```python
from build123d import *

# Parameters (mm, degrees)
SKETCH1_R           = 57.5
SKETCH1_R_2         = 39.25
BOSS_EXTRUDE1_DEPTH = 10
SKETCH2_R           = 1.75
CUT_EXTRUDE1_DEPTH  = 17
SKETCH3_R           = 47
CUT_EXTRUDE2_DEPTH  = 0.75
SKETCH5_R           = 2
CUT_EXTRUDE3_DEPTH  = 5
SKETCH6_R           = 39.25
SKETCH6_R_2         = 35
BOSS_EXTRUDE2_DEPTH = 2


with BuildPart() as part:
    # Sketch1 → Boss-Extrude1 (new body)
    with BuildSketch(Plane(origin=(0, 0, 0), x_dir=(1, 0, 0), z_dir=(0, 1, 0))):
        with Locations(Location((0, 0, 0), (0, 0, 270))):
            Circle(SKETCH1_R)
        with Locations(Location((0, 0, 0), (0, 0, 270))):
            Circle(SKETCH1_R_2, mode=Mode.SUBTRACT)
    extrude(amount=BOSS_EXTRUDE1_DEPTH)

    # Sketch2 → Cut-Extrude1 (cut)
    with BuildSketch(Plane(origin=(0, 10, 0), x_dir=(1, 0, 0), z_dir=(0, 1, 0))):
        with Locations(Location((0, 54, 0), (0, 0, 270))):
            Circle(SKETCH2_R)
        with Locations(Location((20.664905348, 49.889494756, 0), (0, 0, 270))):
            Circle(SKETCH2_R)
        with Locations(Location((38.183766184, 38.183766184, 0), (0, 0, 270))):
            Circle(SKETCH2_R)
        with Locations(Location((49.889494756, 20.664905348, 0), (0, 0, 270))):
            Circle(SKETCH2_R)
        with Locations(Location((54, 0, 0), (0, 0, 270))):
            Circle(SKETCH2_R)
        with Locations(Location((49.889494756, -20.664905348, 0), (0, 0, 270))):
            Circle(SKETCH2_R)
        with Locations(Location((38.183766184, -38.183766184, 0), (0, 0, 270))):
            Circle(SKETCH2_R)
        with Locations(Location((20.664905348, -49.889494756, 0), (0, 0, 270))):
            Circle(SKETCH2_R)
        with Locations(Location((0, -54, 0), (0, 0, 270))):
            Circle(SKETCH2_R)
        with Locations(Location((-20.664905348, -49.889494756, 0), (0, 0, 270))):
            Circle(SKETCH2_R)
        with Locations(Location((-38.183766184, -38.183766184, 0), (0, 0, 270))):
            Circle(SKETCH2_R)
        with Locations(Location((-49.889494756, -20.664905348, 0), (0, 0, 270))):
            Circle(SKETCH2_R)
        with Locations(Location((-54, 0, 0), (0, 0, 270))):
            Circle(SKETCH2_R)
        with Locations(Location((-49.889494756, 20.664905348, 0), (0, 0, 270))):
            Circle(SKETCH2_R)
        with Locations(Location((-38.183766184, 38.183766184, 0), (0, 0, 270))):
            Circle(SKETCH2_R)
        with Locations(Location((-20.664905348, 49.889494756, 0), (0, 0, 270))):
            Circle(SKETCH2_R)
    extrude(amount=-CUT_EXTRUDE1_DEPTH, mode=Mode.SUBTRACT)

    # Sketch3 → Cut-Extrude2 (cut)
    with BuildSketch(Plane(origin=(0, 10, 0), x_dir=(1, 0, 0), z_dir=(0, 1, 0))):
        with Locations(Location((0, 0, 0), (0, 0, 270))):
            Circle(SKETCH3_R)
    extrude(amount=-CUT_EXTRUDE2_DEPTH, mode=Mode.SUBTRACT)

    # Sketch5 → Cut-Extrude3 (cut)
    with BuildSketch(Plane.XZ):
        with Locations(Location((0, 45, 0), (0, 0, 270))):
            Circle(SKETCH5_R)
        with Locations(Location((38.97114317, -22.5, 0), (0, 0, 270))):
            Circle(SKETCH5_R)
        with Locations(Location((-38.97114317, -22.5, 0), (0, 0, 270))):
            Circle(SKETCH5_R)
    extrude(amount=-CUT_EXTRUDE3_DEPTH, mode=Mode.SUBTRACT)

    # Sketch6 → Boss-Extrude2 (add)
    with BuildSketch(Plane.XZ):
        with Locations(Location((0, 0, 0), (0, 0, 270))):
            Circle(SKETCH6_R)
        with Locations(Location((0, 0, 0), (0, 0, 270))):
            Circle(SKETCH6_R_2, mode=Mode.SUBTRACT)
    extrude(amount=-BOSS_EXTRUDE2_DEPTH)


solid = part.part
```
Build history of the part. All positions in model axes, mm. A direction names the side the tool comes from. Round coordinates to 2 decimals unless told otherwise and drop trailing zeros. Loops run counter-clockwise (first coordinate to the right, second up) from the corner with the lowest first, then second, coordinate; pieces in that order, holes last. Notation, with made-up numbers: M -35,68 L 19,68 A20 ccw 19,84 Z; hole C 78,-19.5 d8. An arc over 180 degrees is marked long. Answer as CSV lines item,"result".
1. Wall check: probe 1 along X at (y, z) = (0.6, 0); probe 2 along X at (y, z) = (5, -20); probe 3 along Z at (x, y) = (49.5, 6). Give the ranges that are in metal, low to high. Write a range as [from, to].
Resolved:
probe 1,"x = [-57.5, -55.75], [-52.25, -35], [35, 52.25], [55.75, 57.5]"
probe 2,"x = [-53.91, -51.51], [-48.27, -33.77], [33.77, 48.27], [51.51, 53.91]"
probe 3,"z = [-29.26, -22.37], [-18.96, 18.96], [22.37, 29.26]"
2. Flat gauge pins, fed straight in: P1, Ø6, axis at y = 3.5, z = 21, coming from the +X side; P2, Ø2, axis at y = 1, z = 22, coming from the -X side; P3, Ø3, axis at x = -49.89, z = 20.66, coming from the +Y side; P4, Ø2, axis at y = 9, z = 30, coming from the -X side. Where does each tip first touch, or does it go through?
Resolved:
P1,"stops at x = 54.61"
P2,"stops at x = -53.53"
P3,"passes through"
P4,"stops at x = -49.65"
3. Cut at B-B on z = 32. Write the cut outline in (x, y), then the cut area to 3 significant figures.
Resolved:
outline,"M -47.77,0 L -14.18,0 L -14.18,2 L -22.73,2 L -22.73,9.25 L -34.42,9.25 L -34.42,10 L -47.77,10 Z; M 14.18,0 L 47.77,0 L 47.77,10 L 34.42,10 L 34.42,9.25 L 22.73,9.25 L 22.73,2 L 14.18,2 Z"
area,"518 mm²"
4. Two-plate mould, pull along Z, no slides. Class faces 1 (the cylindrical face through (31.765, 9.63, -34.641)), 2 (the flat face through (-25, 0, -25)), 3 (the cylindrical face through (-56.133, 4.93, -12.465)): released by +Z, released by -Z, zero draft, split by the parting line, or undercut.
Resolved:
face 1,"undercut"
face 2,"zero draft"
face 3,"split by the parting line"
5. Cut at D-D on x = -43.5. Write the cut outline in (y, z).
Resolved:
outline,"M 0,-37.6 L 10,-37.6 L 10,-17.8 L 9.25,-17.8 L 9.25,17.8 L 10,17.8 L 10,37.6 L 0,37.6 Z"
6. Cut at A-A on z = 0. Write the cut outline in (x, y), then the cut area to 3 significant figures.
Resolved:
outline,"M -57.5,0 L -55.75,0 L -55.75,10 L -57.5,10 Z; M -52.25,0 L -35,0 L -35,2 L -39.25,2 L -39.25,9.25 L -47,9.25 L -47,10 L -52.25,10 Z; M 35,0 L 52.25,0 L 52.25,10 L 47,10 L 47,9.25 L 39.25,9.25 L 39.25,2 L 35,2 Z; M 55.75,0 L 57.5,0 L 57.5,10 L 55.75,10 Z"
area,"300 mm²"
7. 3-axis set-ups, long thin cutter, end or side, ignore diameter. For faces 4 (the cylindrical face through (-36.99, 2.46, -22.24)), 5 (the flat face through (-2.7, 2, 35.1)), 6 (the cylindrical face through (50.415, 5.07, 22.334)): which of +Z, -Z, +X, -X, +Y, -Y reach the whole face in a straight line?
Resolved:
face 4,"-Y"
face 5,"+Y"
face 6,"+Y, -Y"
8. Cut at C-C on x = -31. Write the cut outline in (y, z).
Resolved:
outline,"M 0,-48.43 L 10,-48.43 L 10,-35.33 L 9.25,-35.33 L 9.25,-24.07 L 2,-24.07 L 2,-16.25 L 0,-16.25 Z; M 0,16.25 L 2,16.25 L 2,24.07 L 9.25,24.07 L 9.25,35.33 L 10,35.33 L 10,48.43 L 0,48.43 Z"
